from build123d import *

# Parameters (mm, degrees)
SZKIC1_W                    = 40
SZKIC1_H                    = 40
SZKIC1_R                    = 3
DODANIE_WYCI_GNI_CIE1_DEPTH = 3
ZAOKR_GLENIE1_R             = 5


with BuildPart() as part:
    # Szkic1 → Dodanie-wyciągnięcie1 (new body)
    with BuildSketch(Plane.XY):
        with Locations((-6.490790255, 17.411764706)):
            Rectangle(SZKIC1_W, SZKIC1_H)
        with Locations((-16.490790255, 27.411764706)):
            Circle(SZKIC1_R, mode=Mode.SUBTRACT)
        with Locations((3.509209745, 27.411764706)):
            Circle(SZKIC1_R, mode=Mode.SUBTRACT)
        with Locations((-16.490790255, 7.411764706)):
            Circle(SZKIC1_R, mode=Mode.SUBTRACT)
        with Locations((3.509209745, 7.411764706)):
            Circle(SZKIC1_R, mode=Mode.SUBTRACT)
    dodanie_wyci_gni_cie1 = extrude(amount=DODANIE_WYCI_GNI_CIE1_DEPTH)

    # Lustro2: Dodanie-wyciągnięcie1 across plane
    add(dodanie_wyci_gni_cie1.mirror(Plane(origin=(-26.490790255, -2.588235294, 3), x_dir=(0, 0, 1), z_dir=(0, 1, 0))))

    # Zaokrąglenie1
    zaokr_glenie1_edges = [part.edges().sort_by_distance(p)[0] for p in [
        (-26.490790255, -42.588235294, 1.5),
        (13.509209745, -42.588235294, 1.5),
        (-26.490790255, 37.411764706, 1.5),
        (13.509209745, 37.411764706, 1.5),
    ]]
    fillet(zaokr_glenie1_edges, radius=ZAOKR_GLENIE1_R)


solid = part.part
For this review, take the finished solid that the model builds, in its own axes (mm). Round coordinates to 2 decimals unless told otherwise and drop trailing zeros. Order: outer loops, then holes, each group sorted by start corner. A loop starts at its lowest first (then second) coordinate and runs counter-clockwise, first axis right, second up. Notation, with made-up numbers: M 1,-39 L 56,-39 A24 ccw 56,-13 Z; hole C 32,75.25 d4. An arc over 180 degrees is marked long. Use a Markdown table: item, result. Add a question column.
Item 1: Mouldability with a two-part tool opening along X and no side actions: class faces 1 (the flat face through (-26.491, -2, 1)), 2 (the cylindrical face through (1.3, -34.62, 1.48)), 3 (the flat face through (-7, 37.412, 1)) as released by +X, released by -X, zero draft, split by the parting line, or undercut.
Item 2: To check wall thickness, follow line 1 along Y through (x, z) = (1, 1.5); line 2 along X through (y, z) = (29.5, 0.3); line 3 along Y through (x, z) = (2.5, 2.55). State the ranges of each line that lie inside material, in increasing order.
Item 3: Add section C-C, the plane z = 1.25. State how many separate pieces and enclosed holes the cut face has, then the cut area to 3 significant figures.
Item 4: Add section B-B, the plane y = 28.5. Give the boundary of the cut face in (x, z).
Item 5: Add section A-A, the plane x = 3. Give the boundary of the cut face in (y, z).
Geometry results:
| question | item | result |
|---|---|---|
| 1 | face 1 | released by -X |
| 1 | face 2 | undercut |
| 1 | face 3 | zero draft |
| 2 | line 1 | y = -42.59 to -34.23, -30.94 to -14.23, -10.94 to 5.77, 9.06 to 25.77, 29.06 to 37.41 |
| 2 | line 2 | x = -26.49 to -18.64, -14.34 to 1.36, 5.66 to 13.51 |
| 2 | line 3 | y = -42.59 to -35.41, -29.76 to -15.41, -9.76 to 4.59, 10.24 to 24.59, 30.24 to 37.41 |
| 3 | separate pieces | 1 |
| 3 | enclosed holes | 8 |
| 3 | area | 2,950 mm² |
| 4 | outline | M -26.49,0 L -19.29,0 L -19.29,3 L -26.49,3 Z; M -13.7,0 L 0.71,0 L 0.71,3 L -13.7,3 Z; M 6.3,0 L 13.51,0 L 13.51,3 L 6.3,3 Z |
| 5 | outline | M -42.59,0 L -35.54,0 L -35.54,3 L -42.59,3 Z; M -29.63,0 L -15.54,0 L -15.54,3 L -29.63,3 Z; M -9.63,0 L 4.46,0 L 4.46,3 L -9.63,3 Z; M 10.37,0 L 24.46,0 L 24.46,3 L 10.37,3 Z; M 30.37,0 L 37.41,0 L 37.41,3 L 30.37,3 Z |
